```python
from build123d import *

# Parameters (mm, degrees)
SKETCH1_R               = 22.5
SKETCH1_R_2             = 15
BOSS_EXTRUDE1_DEPTH     = 15
SKETCH2_R               = 3
CUT_EXTRUDE1_DEPTH      = 23.5
CUT_EXTRUDE1_DEPTH_BACK = 23.5
FILLET1_R               = 1


with BuildPart() as part:
    # Sketch1 → Boss-Extrude1 (new body)
    with BuildSketch(Plane(origin=(0, 0, 0), x_dir=(1, 0, 0), z_dir=(0, 1, 0))):
        Circle(SKETCH1_R)
        Circle(SKETCH1_R_2, mode=Mode.SUBTRACT)
    extrude(amount=BOSS_EXTRUDE1_DEPTH)

    # Sketch2 → Cut-Extrude1 (cut, two sides)
    with BuildSketch(Plane.XY) as cut_extrude1_sk:
        with Locations((0, 7.5)):
            Circle(SKETCH2_R)
    extrude(amount=CUT_EXTRUDE1_DEPTH, mode=Mode.SUBTRACT)
    extrude(cut_extrude1_sk.sketch, amount=-CUT_EXTRUDE1_DEPTH_BACK, mode=Mode.SUBTRACT)

    # Fillet1
    fillet1_edges = [part.edges().sort_by_distance(p)[0] for p in [
        (-22.5, 0, 0),
        (-22.5, 15, 0),
    ]]
    fillet(fillet1_edges, radius=FILLET1_R)


solid = part.part
```
Model file for the job. Use its own axes, mm. Round coordinates to 2 decimals unless told otherwise and drop trailing zeros. Write each loop counter-clockwise with the first axis right and the second up, starting at its lowest first coordinate (ties: lowest second). Pieces come first, ordered by that corner, then holes. Notation, with made-up numbers: (-39, 26) - (-14, 26) arc R12 ccw to (-14, 30) - close; hole circle Ø7 at (-20, -5.75). An arc over 180 degrees is marked (long way). Use CSV: the item, a comma, the result in double quotes. Start each with the question number.
Item 1: Drill centre lines: L1, parallel to Y at x = 0, z = -18.5; L2, parallel to Z at x = 0, y = 4; L3, parallel to X at y = 7.5, z = 19. Where is each one in solid material? Low to high. Write a range as [from, to].
Item 2: Two-plate mould, pull along Y, no slides. Class faces 1 (the face through (4, 15, -15)), 2 (the face through (-3, 7.6, -18.5)), 3 (the face through (-3, 7.6, 18.5)), 4 (the face through (4, 0, -15)): released by +Y, released by -Y, zero draft, split by the parting line, or undercut.
Item 3: Band-saw the part on C-C (y = 7.5). Write the cut outline in (x, z).
Item 4: Band-saw the part on B-B (z = 0). Write the cut outline in (x, y), and give its area (3 significant figures).
Item 5: Band-saw the part on A-A (x = 0). Write the cut outline in (y, z).
Item 6: Pin check, flat tips, straight feed: P1, Ø5, axis at y = 1.5, z = 12.5, coming from the +X side; P2, Ø8, axis at y = 4, z = -11, coming from the +X side; P3, Ø3.5, axis at x = 0, y = 7.5, coming from the -Z side; P4, Ø2, axis at x = -5, y = 11.5, coming from the +Z side. Stop position of each tip, or through.
Checked values:
1,L1,"y = [0, 4.5], [10.5, 15]"
1,L2,"z = [-22.5, -15], [15, 22.5]"
1,L3,"x = [-12.05, -3], [3, 12.05]"
2,face 1,"released by +Y"
2,face 2,"undercut"
2,face 3,"undercut"
2,face 4,"released by -Y"
3,outline,"(-3, -22.3) - (-3, -14.7) arc R15 cw to (-3, 14.7) - (-3, 22.3) arc R22.5 ccw to start; (3, -22.3) arc R22.5 ccw to (3, 22.3) - (3, 14.7) arc R15 cw to (3, -14.7) - close"
4,outline,"(-22.5, 1) arc R1 ccw to (-21.5, 0) - (-15, 0) - (-15, 15) - (-21.5, 15) arc R1 ccw to (-22.5, 14) - close; (15, 0) - (21.5, 0) arc R1 ccw to (22.5, 1) - (22.5, 14) arc R1 ccw to (21.5, 15) - (15, 15) - close"
4,area,"224 mm²"
5,outline,"(0, -21.5) arc R1 ccw to (1, -22.5) - (4.5, -22.5) - (4.5, -15) - (0, -15) - close; (0, 15) - (4.5, 15) - (4.5, 22.5) - (1, 22.5) arc R1 ccw to (0, 21.5) - close; (10.5, -22.5) - (14, -22.5) arc R1 ccw to (15, -21.5) - (15, -15) - (10.5, -15) - close; (10.5, 15) - (15, 15) - (15, 21.5) arc R1 ccw to (14, 22.5) - (10.5, 22.5) - close"
6,P1,"stops at x = 20.16"
6,P2,"stops at x = 21.38"
6,P3,"passes through"
6,P4,"stops at z = 22.14"
